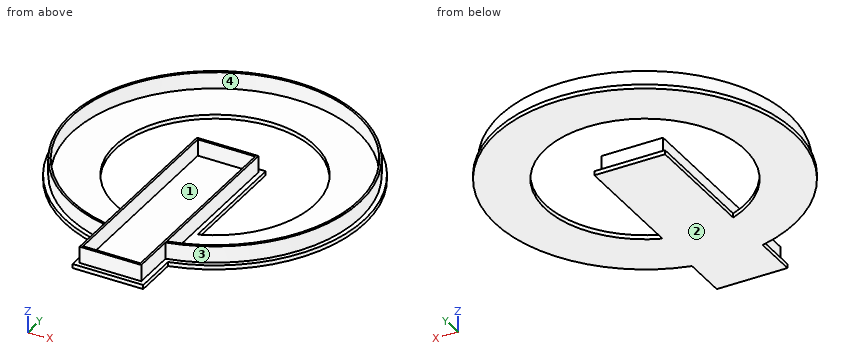
```python
from build123d import *

# Parameters (mm, degrees)
F0_R      = 69.8
F0_R_2    = 68.8
F1_DEPTH  = 10
F2_W      = 29.6
F2_H      = 99.6
F2_W_2    = 27.6
F2_H_2    = 97.6
F3_DEPTH  = 10
F4_R      = 68.8
F4_R_2    = 48
F5_DEPTH  = 2
F6_R      = 72
F6_R_2    = 69.8
F7_DEPTH  = 2
F8_W      = 34
F8_H      = 104
F8_W_2    = 29.6
F8_H_2    = 99.6
F9_DEPTH  = 2
F10_W     = 27.6
F10_H     = 97.6
F11_DEPTH = 2
F12_W     = 27.6
F12_H     = 8
F13_DEPTH = 70


with BuildPart() as f1:
    # F0 (on Top) → F1 (new body)
    with BuildSketch(Plane.XY):
        Circle(F0_R)
        Circle(F0_R_2, mode=Mode.SUBTRACT)
    extrude(amount=F1_DEPTH)

    # F2 (on Top) → F3 (join)
    with BuildSketch(Plane.XY):
        with Locations((0, -39)):
            Rectangle(F2_W, F2_H)
        with Locations((0, -39)):
            Rectangle(F2_W_2, F2_H_2, mode=Mode.SUBTRACT)
    extrude(amount=F3_DEPTH)

    # F4 (on Top) → F5 (join)
    with BuildSketch(Plane.XY):
        Circle(F4_R)
        Circle(F4_R_2, mode=Mode.SUBTRACT)
    extrude(amount=F5_DEPTH)

    # F6 (on Top) → F7 (join)
    with BuildSketch(Plane.XY):
        Circle(F6_R)
        Circle(F6_R_2, mode=Mode.SUBTRACT)
    extrude(amount=F7_DEPTH)

    # F8 (on Top) → F9 (join)
    with BuildSketch(Plane.XY):
        with Locations((0, -39)):
            Rectangle(F8_W, F8_H)
        with Locations((0, -39)):
            Rectangle(F8_W_2, F8_H_2, mode=Mode.SUBTRACT)
    extrude(amount=F9_DEPTH)

    # F10 (on Top) → F11 (join)
    with BuildSketch(Plane.XY):
        with Locations((0, -39)):
            Rectangle(F10_W, F10_H)
    extrude(amount=F11_DEPTH)

    # F12 (on Front) → F13 (cut)
    with BuildSketch(Plane.XZ):
        with Locations((0, 6)):
            Rectangle(F12_W, F12_H)
    extrude(amount=F13_DEPTH, mode=Mode.SUBTRACT)


solid = f1.part
```
Work out the finished part from the listing and answer in its coordinate system (mm). Face numbers are marked on the shaded views. Round coordinates to 2 decimals unless told otherwise and drop trailing zeros. Write each loop counter-clockwise with the first axis right and the second up, starting at its lowest first coordinate (ties: lowest second). Pieces come first, ordered by that corner, then holes.
1) Flat-ended cylindrical pins translate along their axes: P1, Ø2, axis at y = -76.5, z = 1, coming from the +X side; P2, Ø4, axis at x = 25.5, y = -45.5, coming from the +Z side; P3, Ø2.5, axis at y = -81.5, z = 5.5, coming from the +X side. Find the tip coordinate at first contact, or state that the pin passes through.
2) A cutting plane is placed at D-D on x = 20. Determine the outline of the cut face in (y, z), and give its area (3 significant figures).
3) A cutting plane is placed at A-A on y = 0. Determine the outline of the cut face in (x, z), and give its area (3 significant figures).
4) A cutting plane is placed at B-B on z = 7. Determine the outline of the cut face in (x, y), and give its area (3 significant figures).
5) Determine the mould class of the marked faces 1, 2, 3 and 4 for opening direction X: pulls with the +X half, pulls with the -X half, needs draft (parallel to the pull), parting line crosses it, or undercut.
6) Consider probe 1 along X at (y, z) = (0, 5); probe 2 along X at (y, z) = (0, 0.85); probe 3 along Y at (x, z) = (0, 0.65). Determine where each line is inside the solid, lowest interval first.
7) A cutting plane is placed at C-C on x = 0. Determine the outline of the cut face in (y, z), and give its area (3 significant figures).
Entries:
1. P1: stops at x = 17
1. P2: stops at z = 2
1. P3: stops at x = 14.8
2. outline: (-69.17, 0) - (-43.63, 0) - (-43.63, 2) - (-65.83, 2) - (-65.83, 10) - (-66.87, 10) - (-66.87, 2) - (-69.17, 2) - close; (43.63, 0) - (69.17, 0) - (69.17, 2) - (66.87, 2) - (66.87, 10) - (65.83, 10) - (65.83, 2) - (43.63, 2) - close
2. area: 119 mm2
3. outline: (-72, 0) - (-48, 0) - (-48, 2) - (-68.8, 2) - (-68.8, 10) - (-69.8, 10) - (-69.8, 2) - (-72, 2) - close; (-17, 0) - (17, 0) - (17, 2) - (14.8, 2) - (14.8, 10) - (13.8, 10) - (13.8, 2) - (-13.8, 2) - (-13.8, 10) - (-14.8, 10) - (-14.8, 2) - (-17, 2) - close; (48, 0) - (72, 0) - (72, 2) - (69.8, 2) - (69.8, 10) - (68.8, 10) - (68.8, 2) - (48, 2) - close
3. area: 196 mm2
4. outline: (-14.8, -88.8) - (14.8, -88.8) - (14.8, -68.21) arc R69.8 ccw (long way) to (-14.8, -68.21) - close; hole (-14.8, -67.19) - (-14.8, 10.8) - (14.8, 10.8) - (14.8, -67.19) arc R68.8 ccw (long way) to start; hole (-13.8, -87.8) - (13.8, -87.8) - (13.8, 9.8) - (-13.8, 9.8) - close
4. area: 660 mm2
5. face 1: undercut
5. face 2: needs draft
5. face 3: parting line crosses it
5. face 4: undercut
6. probe 1: x = -69.8 to -68.8, -14.8 to -13.8, 13.8 to 14.8, 68.8 to 69.8
6. probe 2: x = -72 to -48, -17 to 17, 48 to 72
6. probe 3: y = -91 to 13, 48 to 72
7. outline: (-91, 0) - (13, 0) - (13, 2) - (10.8, 2) - (10.8, 10) - (9.8, 10) - (9.8, 2) - (-87.8, 2) - (-87.8, 10) - (-88.8, 10) - (-88.8, 2) - (-91, 2) - close; (48, 0) - (72, 0) - (72, 2) - (69.8, 2) - (69.8, 10) - (68.8, 10) - (68.8, 2) - (48, 2) - close
7. area: 280 mm2
